from build123d import *

# Parameters (mm, degrees)
F0_W = 0.8
F0_H = 0.4
F2_R = 0.2
F3_R = 0.3


# Not quite as in the source:
# - a feature names something its author has since deleted; it is built from what else it names


with BuildPart() as f1:
    # F0 (on Front) → F1 (revolve)
    with BuildSketch(Plane.XZ):
        Polygon((-6.35, 0), (0, 0), (0, 1), (-0.8, 1), (-7.35, 1), (-7.35, -0.8), (-6.35, -0.8), align=None)
        with Locations((-0.4, 1.2)):
            Rectangle(F0_W, F0_H)
        with BuildLine():
            Line((-0.8, 1.4), (0, 1.4))
            Line((0, 1.4), (0, 2.2))
            ThreePointArc((0, 2.2), (-0.5656854249, 1.9656854249), (-0.8, 1.4))
        make_face()
    revolve(axis=Axis((0, 0, 0.5), (0, 0, 1)))

    # F2
    f2_edges = [f1.edges().sort_by_distance(p)[0] for p in [
        (7.35, 0, 1),
        (7.35, 0, -0.8),
        (6.35, 0, -0.8),
    ]]
    fillet(f2_edges, radius=F2_R)

    # F3
    f3_edges = [f1.edges().sort_by_distance(p)[0] for p in [
        (0.8, 0, 1),
    ]]
    fillet(f3_edges, radius=F3_R)


solid = f1.part
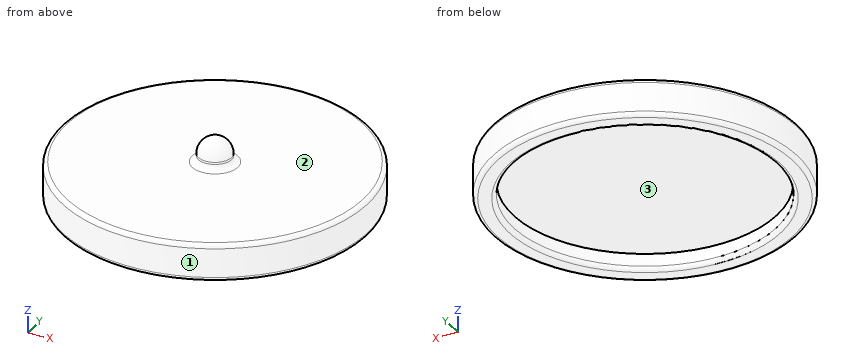
Could you check a few things on this model? Use its own coordinates, in mm. Face numbers are marked on the shaded views. Give positions to 0.01 mm unless a question says otherwise; leave off trailing zeros. Loops run counter-clockwise (first coordinate to the right, second up) from the corner with the lowest first, then second, coordinate; pieces in that order, holes last. Notation, with made-up numbers: (-4, -29) -> (30, -29) arc R17 ccw to (30, -24) -> close; hole circle Ø4 at (75.5, 33.5). An arc over 180 degrees is marked (long way). Return JSON: item names as keys, results as strings.
Item 1: If we section it at C-C on z = -0.3: List the corners of the cut face in (x, y) for me.
Geometry results:
{"outline": "circle Ø14.7 at (0, 0); hole circle Ø12.7 at (0, 0)"}
Item 2: If we section it at A-A on x = 0: List the corners of the cut face in (y, z) for me, plus the area to 3 significant figures.
Geometry results:
{"outline": "(-7.35, -0.6) arc R0.2 ccw to (-7.15, -0.8) -> (-6.55, -0.8) arc R0.2 ccw to (-6.35, -0.6) -> (-6.35, 0) -> (6.35, 0) -> (6.35, -0.6) arc R0.2 ccw to (6.55, -0.8) -> (7.15, -0.8) arc R0.2 ccw to (7.35, -0.6) -> (7.35, 0.8) arc R0.2 ccw to (7.15, 1) -> (1.1, 1) arc R0.3 cw to (0.8, 1.3) -> (0.8, 1.4) arc R0.8 ccw to (-0.8, 1.4) -> (-0.8, 1.3) arc R0.3 cw to (-1.1, 1) -> (-7.15, 1) arc R0.2 ccw to (-7.35, 0.8) -> close", "area": "17.9 mm²"}
Item 3: I'm going to push flat-ended pins straight in: pin 1 (8 mm diameter, centred on x = -5.5, y = -2, fed in from -Z); pin 2 (4.5 mm diameter, centred on x = -3.5, y = 0, fed in from +Z); pin 3 (7.5 mm diameter, centred on x = 0, y = 0, fed in from -Z); pin 4 (1 mm diameter, centred on y = 4.5, z = 1, fed in from +X). Where does each tip first touch, or does it pass through?
Geometry results:
{"pin 1": "stops at z = -0.8", "pin 2": "stops at z = 1", "pin 3": "stops at z = 0", "pin 4": "stops at x = 6.14"}
Item 4: If we section it at D-D on z = 1.6: List the corners of the cut face in (x, y) for me, plus the area to 3 significant figures.
Geometry results:
{"outline": "circle Ø1.55 at (0, 0)", "area": "1.88 mm²"}
Item 5: I need wall thicknesses on L1, parallel to X at y = 0, z = -0.35; L2, parallel to Z at x = 4.75, y = 4.75. Which ranges of each line are inside material? Lowest first, please. Write a range as from..to.
Geometry results:
{"L1": "x = -7.35..-6.35, 6.35..7.35", "L2": "z = -0.8..1"}
Item 6: We'd pull the mould along Y, two halves only. Please class the marked faces 1, 2 and 3: +Y half, -Y half, draft (parallel to the pull), parting line (faces both ways), or undercut.
Geometry results:
{"face 1": "parting line", "face 2": "draft", "face 3": "undercut"}
